from build123d import *

# Parameters (mm, degrees)
SKETCH_1_R               = 2.85
EXTRUDE_1_DEPTH          = 12
SKETCH_2_R               = 2.25
EXTRUDE_2_DEPTH          = 12.5
SKETCH_3_R               = 2
CUT_EXTRUDE_1_DEPTH      = 12
CHAMFER_1_SIZE           = 1.5
CHAMFER_1_SIZE2          = 0.545955351
CUT_EXTRUDE_2_DEPTH      = 25.829317349
CUT_EXTRUDE_2_DEPTH_BACK = 25.829317349
SKETCH_4_W               = 6.375471686
SKETCH_4_H               = 4.193701662
SKETCH_5_W               = 0.7
SKETCH_5_H               = 0.3
CHAMFER_2_SIZE           = 0.6
CHAMFER_2_SIZE_2         = 1.039230485
SKETCH_6_W               = 0.6
SKETCH_6_H               = 5
SKETCH_6_W_2             = 5
SKETCH_6_H_2             = 0.6
CUT_EXTRUDE_3_DEPTH      = 10.5
FILLET_1_SIZE            = 1
FILLET_1_SIZE_2          = 0.5


with BuildPart() as part:
    # Эскиз1 → Бобышка-Вытянуть1 (new body)
    with BuildSketch(Plane.XY):
        Circle(SKETCH_1_R)
    extrude(amount=EXTRUDE_1_DEPTH)

    # Эскиз2 → Бобышка-Вытянуть2 (add)
    with BuildSketch(Plane.XY.offset(12)):
        Circle(SKETCH_2_R)
    extrude(amount=EXTRUDE_2_DEPTH)

    # Эскиз3 → Вырез-Вытянуть1 (cut)
    with BuildSketch(Plane(origin=(0, 0, 0), x_dir=(-1, 0, 0), z_dir=(0, 0, -1))):
        Circle(SKETCH_3_R)
    extrude(amount=-CUT_EXTRUDE_1_DEPTH, mode=Mode.SUBTRACT)

    # Фаска1
    chamfer_1_edges = [part.edges().sort_by_distance(p)[0] for p in [
        (2, 0, 12),
    ]]
    chamfer_1_side = [part.faces().sort_by_distance(p)[0] for p in [
        (0, 0, 12),
    ]]
    chamfer(chamfer_1_edges, length=CHAMFER_1_SIZE, length2=CHAMFER_1_SIZE2, reference=chamfer_1_side[0])

    # Эскиз4 → Вырез-Вытянуть2 (cut, two sides: drawn at the far end of the back side and taken through both)
    with BuildSketch(Plane(origin=(0, 0, 0), x_dir=(0, 0, -1), z_dir=(1, 0, 0)).offset(-CUT_EXTRUDE_2_DEPTH_BACK)):
        with Locations((-0.812264157, 2.096850831)):
            Rectangle(SKETCH_4_W, SKETCH_4_H)
    extrude(amount=CUT_EXTRUDE_2_DEPTH + CUT_EXTRUDE_2_DEPTH_BACK, mode=Mode.SUBTRACT)

    # Эскиз5 → Вырез-Повернуть1 (revolve, cut)
    with BuildSketch(Plane(origin=(0, 0, 0), x_dir=(0, 0, -1), z_dir=(1, 0, 0))):
        with Locations((-3.45, -2.85)):
            Rectangle(SKETCH_5_W, SKETCH_5_H)
        with Locations((-2.25, -2.85)):
            Rectangle(SKETCH_5_W, SKETCH_5_H)
        with Locations((-1.05, -2.85)):
            Rectangle(SKETCH_5_W, SKETCH_5_H)
    revolve(axis=Axis((0, 0, 0), (0, 0, 1)), mode=Mode.SUBTRACT)

    # Фаска2
    # the kernel refuses this chamfer: 1.039230485, 0.6 mm, written as the material it adds along each edge
    with BuildSketch(Plane(origin=(0, 0, 12), x_dir=(1, 0, 0), z_dir=(0, -1, 0))) as chamfer_2_piece_1_section:
        Polygon((2.25 + CHAMFER_2_SIZE, 0), (2.25, CHAMFER_2_SIZE_2), (2.25, 0), align=None)
    chamfer_2_piece_1 = revolve(axis=Axis((0, 0, 12), (0, 0, 1)), mode=Mode.PRIVATE)
    chamfer_2_piece_1 = chamfer_2_piece_1 & Plane(origin=(0, 0, 12.528833644), x_dir=(1, 0, 0), z_dir=(0, 0, -1)) * Cylinder(2.85, 12, mode=Mode.PRIVATE)
    add(chamfer_2_piece_1)

    # Эскиз6 → Вырез-Вытянуть3 (cut)
    with BuildSketch(Plane.XY.offset(24.5)):
        Rectangle(SKETCH_6_W, SKETCH_6_H)
        Rectangle(SKETCH_6_W_2, SKETCH_6_H_2)
    extrude(amount=-CUT_EXTRUDE_3_DEPTH, mode=Mode.SUBTRACT)

    # Скругление1
    # an asymmetric fillet: 1, 0.5 mm, written as the material it takes off along each edge
    with BuildSketch(Plane(origin=(0, 0, 24.5), x_dir=(0.8292066330076089, 0.5589421792781295, 0), z_dir=(0.5589421792781295, -0.8292066330076089, 0))) as fillet_1_piece_1:
        with BuildLine():
            Bezier((2.25, -FILLET_1_SIZE), (2.25, 0), (2.25 - FILLET_1_SIZE_2, 0), weights=[1, 0.707106781, 1])
            Line((2.25 - FILLET_1_SIZE_2, 0), (2.25, 0))
            Line((2.25, 0), (2.25, -FILLET_1_SIZE))
        make_face()
    revolve(axis=Axis((0, 0, 24.5), (0, 0, 1)), revolution_arc=202.034652165, mode=Mode.SUBTRACT)
    with BuildSketch(Plane(origin=(0, 0, 24.5), x_dir=(-0.5589421792781271, 0.8292066330076105, 0), z_dir=(0.8292066330076105, 0.5589421792781271, 0))) as fillet_1_piece_2:
        with BuildLine():
            Bezier((2.25, -FILLET_1_SIZE), (2.25, 0), (2.25 - FILLET_1_SIZE_2, 0), weights=[1, 0.707106781, 1])
            Line((2.25 - FILLET_1_SIZE_2, 0), (2.25, 0))
            Line((2.25, 0), (2.25, -FILLET_1_SIZE))
        make_face()
    revolve(axis=Axis((0, 0, 24.5), (0, 0, 1)), revolution_arc=202.034652165, mode=Mode.SUBTRACT)
    with BuildSketch(Plane(origin=(0, 0, 24.5), x_dir=(-0.8292066330076107, -0.5589421792781271, 0), z_dir=(-0.5589421792781271, 0.8292066330076107, 0))) as fillet_1_piece_3:
        with BuildLine():
            Bezier((2.25, -FILLET_1_SIZE), (2.25, 0), (2.25 - FILLET_1_SIZE_2, 0), weights=[1, 0.707106781, 1])
            Line((2.25 - FILLET_1_SIZE_2, 0), (2.25, 0))
            Line((2.25, 0), (2.25, -FILLET_1_SIZE))
        make_face()
    revolve(axis=Axis((0, 0, 24.5), (0, 0, 1)), revolution_arc=202.034652165, mode=Mode.SUBTRACT)
    with BuildSketch(Plane(origin=(0, 0, 24.5), x_dir=(0.5589421792781443, -0.8292066330075989, 0), z_dir=(-0.8292066330075989, -0.5589421792781443, 0))) as fillet_1_piece_4:
        with BuildLine():
            Bezier((2.25, -FILLET_1_SIZE), (2.25, 0), (2.25 - FILLET_1_SIZE_2, 0), weights=[1, 0.707106781, 1])
            Line((2.25 - FILLET_1_SIZE_2, 0), (2.25, 0))
            Line((2.25, 0), (2.25, -FILLET_1_SIZE))
        make_face()
    revolve(axis=Axis((0, 0, 24.5), (0, 0, 1)), revolution_arc=202.034652165, mode=Mode.SUBTRACT)


solid = part.part
Work out the finished part from the listing and answer in its coordinate system (mm). A direction names the side the tool comes from. Give positions to 0.01 mm unless a question says otherwise; leave off trailing zeros. Loops run counter-clockwise (first coordinate to the right, second up) from the corner with the lowest first, then second, coordinate; pieces in that order, holes last. Notation, with made-up numbers: (50, 23) - (76, 23) arc R19 ccw to (76, 27) - close; hole circle Ø10 at (59.25, 4.25). An arc over 180 degrees is marked (long way). Answer in a Markdown table with one row per item. Add a question column.
Q1. The part is cut by section B-B (x = 0). Determine the outline of the cut face in (y, z), and give its area (3 significant figures).
Q2. The part is cut by section C-C (z = 4.75). Determine the outline of the cut face in (x, y), and give its area (3 significant figures).
Q3. Determine the mould class of faces 1 (the flat face through (1, 1, 24.5)), 2 (the cylindrical face through (-0.1, -2.7, 3.4)), 3 (the flat face through (0.3, 1, 19)) for opening direction Z: released by +Z, released by -Z, zero draft, split by the parting line, or undercut.
Q4. A tool of negligible diameter and unlimited length cuts with its end or side. For faces 4 (the flat face through (2.4, 0, 2)), 5 (the flat face through (-0.3, 1, 19)), 6 (the cylindrical face through (-0.06, -2.85, 0.35)), 7 (the flat face through (1, 0.3, 19)), 8 (the cylindrical face through (2.08, -0.86, 18.2)), from which of +Z, -Z, +X, -X, +Y, -Y can it reach the whole face along a straight path? Write none if from no direction.
Q5. Consider line 1 along Y through (x, z) = (0.15, 7); line 2 along Y through (x, z) = (1.45, 22.25); line 3 along X through (y, z) = (0, 5). Determine where each line is inside the solid, lowest interval first.
Q6. Each of these flat-tipped pins is pushed along its axis until it touches: P1, Ø2, axis at x = 1.5, z = 17, coming from the +Y side; P2, Ø0.6, axis at y = -1, z = 18.5, coming from the +X side; P3, Ø2, axis at y = 0, z = 20, coming from the +X side. Where does it stop, or does it pass through?
Q7. The part is cut by section A-A (z = 21). Determine the outline of the cut face in (x, y).
Solution:
| question | item | result |
|---|---|---|
| 1 | outline | (-2.85, 0) - (-2, 0) - (-2, 11.45) - (-0.5, 12) - (0.5, 12) - (2, 11.45) - (2, 4) - (2.85, 4) - (2.85, 12) - (2.25, 13.04) - (2.25, 14) - (-2.25, 14) - (-2.25, 13.04) - (-2.85, 12) - (-2.85, 3.8) - (-2.7, 3.8) - (-2.7, 3.1) - (-2.85, 3.1) - (-2.85, 2.6) - (-2.7, 2.6) - (-2.7, 1.9) - (-2.85, 1.9) - (-2.85, 1.4) - (-2.7, 1.4) - (-2.7, 0.7) - (-2.85, 0.7) - close |
| 1 | area | 27.1 mm² |
| 2 | outline | circle Ø5.7 at (0, 0); hole circle Ø4 at (0, 0) |
| 2 | area | 13.0 mm² |
| 3 | face 1 | released by +Z |
| 3 | face 2 | undercut |
| 3 | face 3 | zero draft |
| 4 | face 4 | -Z, +X, -X, +Y |
| 4 | face 5 | +Z, +Y, -Y |
| 4 | face 6 | +Z, -Z, -Y |
| 4 | face 7 | +Z, +X, -X |
| 4 | face 8 | +Z |
| 5 | line 1 | y = -2.85 to -1.99, 1.99 to 2.85 |
| 5 | line 2 | y = -1.72 to -0.3, 0.3 to 1.72 |
| 5 | line 3 | x = -2.85 to -2, 2 to 2.85 |
| 6 | P1 | stops at y = 2.19 |
| 6 | P2 | stops at x = 2.14 |
| 6 | P3 | stops at x = 2.23 |
| 7 | outline | (-2.23, -0.3) arc R2.25 ccw to (-0.3, -2.23) - (-0.3, -0.3) - close; (-2.23, 0.3) - (-0.3, 0.3) - (-0.3, 2.23) arc R2.25 ccw to start; (0.3, -2.23) arc R2.25 ccw to (2.23, -0.3) - (0.3, -0.3) - close; (0.3, 0.3) - (2.23, 0.3) arc R2.25 ccw to (0.3, 2.23) - close |
